Autodesk Inventor part; units mm, degrees
ref_plane "YZ Plane" through (0, 0, 0) normal (1, 0, 0) x (0, 1, 0)
ref_plane "XZ Plane" through (0, 0, 0) normal (0, 1, 0) x (-1, 0, 0)
ref_plane "XY Plane" through (0, 0, 0) normal (0, 0, 1) x (1, 0, 0)
sketch "Sketch1" plane through (0, 0, 0) normal (0, 1, 0) x (-1, 0, 0)
  line L0 (25, 100) -> (-25, 100)
  line L1 (-25, 100) -> (-25, -100)
  line L2 (-25, -100) -> (25, -100)
  line L3 (25, -100) -> (25, 100)
  line L4 (25, 100) -> (-25, -100) construction
  line L5 (-25, 100) -> (25, -100) construction
  point P0 (0, 0)
  dimension "d0" = 200
  dimension "d1" = 50
extrude "Extrusion1" add sketch "Sketch1" along normal blind 5
sketch "Sketch2" plane through (0, 5, 0) normal (0, 1, 0) x (1, 0, 0)
  line L0 (0, 0) -> (25, 0) construction
  line L1 (25, -100) -> (25, 100)
  line L2 (25, -92) -> (-15.0756, -92) construction
  circle A0 centre (17.5, -92) radius 2
  circle A1 centre (5.5, -92) radius 2
  line L3 (-25, -100) -> (25, -100)
  circle A2 centre (17.5, 92) radius 2
  circle A3 centre (5.5, 92) radius 2
  dimension "d4" = 4
  dimension "d5" = 4
  dimension "d6" = 12
  dimension "d7" = 8
  dimension "d10" = 7.5
extrude "Extrusion2" cut sketch "Sketch2" against normal blind 5
sketch "Sketch3" plane through (0, 5, 0) normal (0, 1, 0) x (1, 0, 0)
  line L0 (19, -85) -> (31, -85)
  line L1 (31, -85) -> (31, 85)
  line L2 (31, 85) -> (19, 85)
  line L3 (19, 85) -> (19, -85)
  line L4 (25, -100) -> (25, 100)
  line L5 (19, -85) -> (31, 85) construction
  line L6 (31, -85) -> (19, 85) construction
  point P0 (0, 0)
  point P1 (25, 0)
  dimension "d11" = 170
  dimension "d12" = 12
extrude "Extrusion3" add sketch "Sketch3" against normal blind 5
sketch "Sketch4" plane through (0, 5, 0) normal (0, 1, 0) x (1, 0, 0)
  line L0 (25, -100) -> (25, -85)
  line L1 (31, 85) -> (25, 85)
  circle A0 centre (26, -75) radius 2
  line L2 (25, -85) -> (31, -85)
  line L3 (31, -85) -> (31, 85)
  point P0 (0, 0)
  dimension "d15" = 4
  dimension "d16" = 10
  dimension "d17" = 5
extrude "Extrusion4" cut sketch "Sketch4" against normal blind 5
pattern_linear "Rectangular Pattern1" count 6 spacing 30 along (0, 0, -1) of "Extrusion4"
fillet "Fillet1" radius 10 2 edges at (-25, 2.5, -100) (-25, 2.5, 100)
sketch "Sketch5" plane through (0, 5, 0) normal (0, 1, 0) x (1, 0, 0)
  line L0 (29.0333, 88) -> (31, 85)
  line L1 (29.0333, 88) -> (-29, 88)
  line L2 (-29, 88) -> (-29, -105)
  line L3 (-29, -105) -> (31, -105)
  line L4 (31, -105) -> (31, 85)
  line L5 (25, 100) -> (-15, 100)
  point P0 (0, 0)
  point P1 (25, 85)
  dimension "d26" = 12
extrude "Extrusion5" cut sketch "Sketch5" against normal blind 10
properties part number "Comb3"
Can you work these out from the model? Positions are in its coordinate system, mm. Give positions to 0.01 mm unless a question says otherwise; leave off trailing zeros. Loops run counter-clockwise (first coordinate to the right, second up) from the corner with the lowest first, then second, coordinate; pieces in that order, holes last. Notation, with made-up numbers: M 56,51.5 L 112,51.5 A21 ccw 112,73.5 Z; hole C -1,31.5 d5. An arc over 180 degrees is marked long. Use one line per item in the form item = value. Start each with the question number.
(1) I want a section at D-D, the plane z = -96.5. Write out the boundary of the cut face in (x, y).
(2) I want a section at C-C, the plane z = -91. Write out the boundary of the cut face in (x, y), and give its area (3 significant figures).
(3) I'm going to push a flat-ended pin straight in: P1, Ø1, axis at x = -20, y = 2.5, coming from the -Z side. Where does the tip first touch, or does it pass through?
(4) Thinking about a two-plate mould opening in Z: for faces 1 (the cylindrical face through (-21.99, 2.54, -97.15)), 2 (the flat face through (0, 5, -94)), 3 (the cylindrical face through (17.24, 2.535, -93.983)), which applies, released by +Z, released by -Z, zero draft, split by the parting line, or undercut?
(5) I want a section at B-B, the plane y = 3.2. Write out the boundary of the cut face in (x, z), and give its area (3 significant figures).
(6) I want a section at A-A, the plane x = 5.5. Write out the boundary of the cut face in (y, z), and give its area (3 significant figures).
(7) Please list where these lines run through material, in increasing order: line 1 (Z direction, x = 5.5, y = 3.75); line 2 (X direction, y = 3, z = -92.5); line 3 (X direction, y = 3.9, z = -92).
Worked out:
q1.outline = M -22.6,0 L 25,0 L 25,5 L -22.6,5 Z
q2.outline = M -24.95,0 L 3.77,0 L 3.77,5 L -24.95,5 Z; M 7.23,0 L 15.77,0 L 15.77,5 L 7.23,5 Z; M 19.23,0 L 25,0 L 25,5 L 19.23,5 Z
q2.area = 215 mm²
q3.P1 = -98.93
q4.face_1 = released by -Z
q4.face_2 = zero draft
q4.face_3 = undercut
q5.outline = M -25,-90 A10 ccw -15,-100 L 25,-100 L 25,-88 L -25,-88 Z; hole C 5.5,-92 d4; hole C 17.5,-92 d4
q5.area = 553 mm²
q6.outline = M 0,-100 L 5,-100 L 5,-94 L 0,-94 Z; M 0,-90 L 5,-90 L 5,-88 L 0,-88 Z
q6.area = 40.0 mm²
q7.line_1 = -100 to -94, -90 to -88
q7.line_2 = -24.68 to 3.56, 7.44 to 15.56, 19.44 to 25
q7.line_3 = -24.8 to 3.5, 7.5 to 15.5, 19.5 to 25
